Verification items for the finished model (mm, model axes). A direction names the side the tool comes from. Coordinates: 2 decimals unless noted, no trailing zeros. Order: outer loops, then holes, each group sorted by start corner. A loop starts at its lowest first (then second) coordinate and runs counter-clockwise, first axis right, second up. Notation, with made-up numbers: M 76.25,-20 L 119.25,-20 A20 ccw 119.25,1 Z; hole C -33.75,21 d9. An arc over 180 degrees is marked long. Write item = value, one per line.
Autodesk Fusion 360 part; units mm, degrees
sketch "mainBase" plane through (0, 0, 0) normal (0, 0, 1) x (1, 0, 0)
  line L0 (0, 0) -> (13.7, 0)
  line L1 (13.7, 0) -> (13.7, 6)
  line L2 (13.7, 6) -> (0, 6)
  line L3 (0, 6) -> (0, 0)
  line L4 (0, 0) -> (6.85, 0)
  line L5 (6.85, 0) -> (6.85, 1.75)
  line L6 (6.85, 1.75) -> (1.85, 1.75)
  line L7 (6.85, 1.75) -> (11.85, 1.75)
  line L8 (0, 6) -> (6.85, 6)
  circle A0 centre (1.85, 1.75) radius 1
  circle A1 centre (11.85, 1.75) radius 1
  line L9 (6.85, 6) -> (3.35, 6)
  line L10 (3.35, 6) -> (3.35, 2)
  line L11 (3.35, 2) -> (6.85, 2)
  line L12 (6.85, 2) -> (6.85, 6)
  line L13 (6.85, 6) -> (10.35, 6)
  line L14 (10.35, 6) -> (10.35, 2)
  line L15 (10.35, 2) -> (6.85, 2)
  line L16 (6.85, 2) -> (6.85, 6)
  dimension "d9" = 6
  dimension "d10" = 13.7
  dimension "d11" = 6.85
  dimension "d12" = 1.75
  dimension "d13" = 5
  dimension "d14" = 5
  dimension "d15" = 6.85
  dimension "d17" = 2
  dimension "d18" = 2
  dimension "d19" = 4
  dimension "d20" = 3.5
  dimension "d21" = 4
  dimension "d22" = 3.5
extrude "Extrude1" add sketch "mainBase" along normal blind 7.6 contours L2 L8 L9 L10 L11 L12 L16 | L2 L12 L13 L14 L15 L16
shell "Shell1" thickness 1 removed faces 1 at (5.6833, 4.6667, 0)
extrude "Extrude2" add sketch "mainBase" along normal blind 2 contours L0 L1 L2 L3 L4 L8 L10 L11 L14 L15
sketch "hallCutOut" plane through (0, 0, 0) normal (0, 0, 1) x (1, 0, 0)
  line L0 (0, 6) -> (6.85, 6)
  line L1 (6.85, 6) -> (6.85, 2)
  line L2 (6.85, 2) -> (3.35, 2)
  line L3 (3.35, 2) -> (3.35, 4)
  line L4 (6.85, 2) -> (6.85, 3)
  line L5 (6.85, 3) -> (5.95, 3)
  line L6 (5.95, 3) -> (3.35, 4)
  line L7 (6.85, 3) -> (7.75, 3)
  line L8 (6.85, 2) -> (10.35, 2)
  line L9 (10.35, 2) -> (10.35, 4)
  line L10 (10.35, 4) -> (7.75, 3)
  line L11 (7.75, 3) -> (9.35, 3)
  line L12 (9.35, 3) -> (9.35, 3.6154)
  line L13 (5.95, 3) -> (4.35, 3)
  line L14 (4.35, 3) -> (4.35, 3.6154)
  line L15 (6.85, 5) -> (8.95, 5)
  line L16 (8.95, 5) -> (8.95, 3)
  line L17 (8.95, 3) -> (6.85, 3)
  line L18 (6.85, 3) -> (6.85, 5)
  line L19 (6.85, 5) -> (4.75, 5)
  line L20 (4.75, 5) -> (4.75, 3)
  line L21 (4.75, 3) -> (6.85, 3)
  line L22 (6.85, 3) -> (6.85, 5)
  line L23 (9.35, 3) -> (4.35, 3)
  line L24 (4.35, 3) -> (4.35, 5)
  line L25 (4.35, 5) -> (9.35, 5)
  line L26 (9.35, 5) -> (9.35, 3)
  dimension "d31" = 6.85
  dimension "d32" = 4
  dimension "d33" = 3.5
  dimension "d34" = 2
  dimension "d35" = 1
  dimension "d36" = 0.9
  dimension "d37" = 0.9
  dimension "d38" = 3.5
  dimension "d39" = 2
  dimension "d59" = 2.1
extrude "Extrude3" add sketch "hallCutOut" along normal blind 6.6 contours L6 L13 L20 L21 L23 | L10 L11 L16 L17 L23 | L10 L11 L12 L16 L23 L26 | L6 L13 L14 L20 L23 L24
sketch "wireCutOut" plane through (0, 0, 0) normal (0, -1, 0) x (1, 0, 0)
  line L0 (0, 0) -> (13.7, 0)
  line L1 (13.7, 0) -> (13.7, 2)
  line L2 (13.7, 2) -> (0, 2)
  line L3 (0, 2) -> (0, 0)
  line L4 (0, 0) -> (6.85, 0)
  line L5 (6.85, 0) -> (6.85, 1)
  line L6 (6.85, 1) -> (5.95, 1)
  line L7 (6.85, 1) -> (7.75, 1)
  line L8 (6.85, 0) -> (13.7, 0)
  line L9 (6.85, 0) -> (10.35, 0)
  line L10 (6.85, 0) -> (3.35, 0)
  line L11 (7.75, 1) -> (10.35, 0)
  line L12 (5.95, 1) -> (3.35, 0)
  dimension "d42" = 6.85
  dimension "d43" = 1
  dimension "d44" = 0.9
  dimension "d45" = 0.9
  dimension "d46" = 6.85
  dimension "d47" = 3.5
  dimension "d48" = 3.5
extrude "Extrude4" cut sketch "wireCutOut" against normal blind 5 contours L0 L4 L5 L6 L10 L12 | L0 L5 L7 L8 L9 L11
sketch "cutOut" plane through (0, 0, 0) normal (0, 0, 1) x (1, 0, 0)
  line L0 (0, 0) -> (13.7, 0)
  line L1 (13.7, 0) -> (13.7, 6)
  line L2 (13.7, 6) -> (0, 6)
  line L3 (0, 6) -> (0, 0)
  line L4 (13.7, 0) -> (13.7, 2)
  line L5 (0, 0) -> (0, 2)
  line L6 (0, 6) -> (2, 6)
  line L7 (13.7, 6) -> (11.7, 6)
  line L8 (0, 2) -> (2, 6)
  line L9 (13.7, 2) -> (11.7, 6)
  dimension "d51" = 6
  dimension "d52" = 13.7
  dimension "d53" = 2
  dimension "d54" = 2
  dimension "d55" = 2
  dimension "d56" = 2
extrude "Extrude5" cut sketch "cutOut" along normal blind 2 contours L2 L3 L6 L8 | L1 L2 L7 L9
extrude "Extrude6" add sketch "hallCutOut" along normal blind 7.6 contours L10 L16 L25 L26 | L6 L20 L24 L25
extrude "Extrude7" cut sketch "wireCutOut" against normal blind 5 contours L0 L4 L5 L6 L10 L12 | L0 L5 L7 L8 L9 L11
equation "baseLength = 6 mm"
equation "baseWidth = 13.7 mm"
equation "mountingCircleToMountingCircle = 10 mm"
equation "mountingHoleFromEdge = 1.75 mm"
equation "hallEffectWidth = 7 mm"
equation "hallEffectLength = 4 mm"
equation "hallEffectHeight = 7.6 mm"
equation "baseHeight = 2 mm"
equation "d9 = baseLength"
equation "d10 = baseWidth"
equation "d11 = baseWidth / 2"
equation "d12 = mountingHoleFromEdge"
equation "d13 = mountingCircleToMountingCircle / 2"
equation "d14 = mountingCircleToMountingCircle / 2"
equation "d15 = baseWidth / 2"
equation "screwHole = 2 mm"
equation "d17 = screwHole"
equation "d18 = screwHole"
equation "d19 = hallEffectLength"
equation "d20 = hallEffectWidth / 2"
equation "d21 = hallEffectLength"
equation "d22 = hallEffectWidth / 2"
equation "d23 = hallEffectHeight"
equation "hallEffectThickness = 1 mm"
equation "d26 = hallEffectThickness"
equation "d27 = baseHeight"
equation "traingleHeight = 2 mm"
equation "hallEffectMiddleDist = 1.8 mm"
equation "d31 = baseWidth / 2"
equation "d32 = hallEffectLength"
equation "d33 = hallEffectWidth / 2"
equation "d34 = traingleHeight"
equation "d35 = hallEffectThickness"
equation "d36 = hallEffectMiddleDist / 2"
equation "d37 = hallEffectMiddleDist / 2"
equation "d38 = hallEffectWidth / 2"
equation "d39 = traingleHeight"
equation "d40 = hallEffectHeight - hallEffectThickness"
equation "d42 = baseWidth / 2"
equation "d43 = hallEffectThickness"
equation "d44 = hallEffectMiddleDist / 2"
equation "d45 = hallEffectMiddleDist / 2"
equation "d46 = baseWidth / 2"
equation "d47 = hallEffectWidth / 2"
equation "d48 = hallEffectWidth / 2"
equation "d51 = baseLength"
equation "d52 = baseWidth"
equation "d53 = baseLength / 3"
equation "d54 = baseLength / 3"
equation "d57 = baseHeight"
equation "d60 = hallEffectHeight"
Item 1: Gauge pin test, flat ends, axial feed: pin 1 (0.8 mm diameter, centred on y = 4, z = 4.5, fed in from +X); pin 2 (1.4 mm diameter, centred on x = 7, y = 1.5, fed in from -Z); pin 3 (1.5 mm diameter, centred on y = 2.5, z = 6.5, fed in from -X). Record the tip position at first contact, or that the pin passes through.
Report:
pin_1 = 10.35
pin_2 = 1
pin_3 = 3.35
Item 2: Sectioned sample at C-C, the plane z = 1.25. Enter the section's corners in (x, y).
Report:
outline = M 0,0 L 13.7,0 L 13.7,2 L 11.7,6 L 2,6 L 0,2 Z; hole C 1.85,1.75 d2; hole M 4.75,3.46 L 5.95,3 L 7.75,3 L 8.95,3.46 L 8.95,5 L 4.75,5 Z; hole C 11.85,1.75 d2
Item 3: Sectioned sample at D-D, the plane z = 5.5. Enter the section's corners in (x, y), then the cut area to 3 significant figures.
Report:
outline = M 3.35,2 L 10.35,2 L 10.35,6 L 3.35,6 Z; hole M 4.75,3.46 L 5.95,3 L 7.75,3 L 8.95,3.46 L 8.95,5 L 4.75,5 Z
area = 20.2 mm^2
Item 4: Release check for a two-part mould opening along X. For faces 1 (the flat face through (8.358, 3.234, 3.527)), 2 (the flat face through (7, 6, 4)), 3 (the flat face through (1, 4, 1)) record: pulls with the +X half, pulls with the -X half, needs draft (parallel to the pull), parting line crosses it, or undercut.
Report:
face_1 = undercut
face_2 = needs draft
face_3 = pulls with the -X half
Item 5: Scan lines: L1, parallel to X at y = 3.7, z = 6.25; L2, parallel to Z at x = 1.25, y = 0.8; L3, parallel to Y at x = 9, z = 5.75. Record each from-to range of solid material in increasing order. Write a range as from..to.
Report:
L1 = 3.35..4.75, 8.95..10.35
L2 = 0..2
L3 = 2..6
Item 6: Sectioned sample at B-B, the plane x = 11.85. Enter the section's corners in (y, z), then the cut area to 3 significant figures.
Report:
outline = M 0,0 L 0.75,0 L 0.75,2 L 0,2 Z; M 2.75,0 L 5.7,0 L 5.7,2 L 2.75,2 Z
area = 7.40 mm^2
Item 7: Tool access check on faces 4 (the flat face through (3.35, 4, 5)), 5 (the flat face through (7, 2, 5)), 6 (the flat face through (7, 1, 1)), 7 (the flat face through (5.358, 3.228, 3.527)), 8 (the flat face through (10.35, 4, 5)). Record the directions out of +Z, -Z, +X, -X, +Y, -Y that give a thin tool (end or side, any length) a straight path to the whole face; none if there is none.
Report:
face_4 = +Z, -X, +Y, -Y
face_5 = +Z, +X, -X, -Y
face_6 = -Z, -Y
face_7 = -Z
face_8 = +Z, +X, +Y, -Y
Item 8: Sectioned sample at A-A, the plane y = 1.75. Enter the section's corners in (x, z).
Report:
outline = M 0,0 L 0.85,0 L 0.85,2 L 0,2 Z; M 2.85,0 L 3.35,0 L 5.95,1 L 7.75,1 L 10.35,0 L 10.85,0 L 10.85,2 L 2.85,2 Z; M 12.85,0 L 13.7,0 L 13.7,2 L 12.85,2 Z
